from build123d import *

# Parameters (mm, degrees)
F4_T = -10
F5_R = 10


with BuildPart() as f3:
    # F0 (on Top) → F3 section 0
    with BuildSketch(Plane.XY):
        Polygon((19.5, 0), (0, 0), (-19.5, 0), (-35, -68.2623615179), (0, -68.2623615179), (35, -68.2623615179), align=None)
    # F2 (on offset) → F3 section 1
    with BuildSketch(Plane.XY.offset(-50)):
        Polygon((0, -83.2623615179), (53.7878059224, -83.2623615179), (31.4758528979, 15), (0, 15), (-31.4758528979, 15), (-53.7878059224, -83.2623615179), align=None)
    loft()

    # F4
    f4_openings = [f3.faces().sort_by_distance(p)[0] for p in [
        (0, -37.366858, 0),
        (0, -38.41676, -50),
    ]]
    offset(amount=F4_T, openings=f4_openings, kind=Kind.INTERSECTION)

    # F5
    f5_edges = [f3.edges().sort_by_distance(p)[0] for p in [
        (-25.487926, 7.5, -25),
        (-44.393903, -75.762362, -25),
        (44.393903, -75.762362, -25),
        (25.487926, 7.5, -25),
    ]]
    fillet(f5_edges, radius=F5_R)


solid = f3.part
Input: part model. Units: mm. Frame: model coordinates. A direction names the side the tool comes from. Round coordinates to 2 decimals unless told otherwise and drop trailing zeros.
1. Set-up query: faces 1 (the face through (-0.57, -67.094, -30.906)), 2 (the face through (33, -34, -50)). Return all of +Z, -Z, +X, -X, +Y, -Y with unobstructed straight access to the full face (end or side cutting, diameter ignored); none if empty.
The answers:
face 1: -Z
face 2: -Z, +X, -X, +Y, -Y
2. Pin query (flat end, axial travel): P1, Ø8, axis at x = 24.5, z = -14, coming from the +Y side; P2, Ø1, axis at y = -42, z = -23.5, coming from the -X side; P3, Ø1, axis at y = -44, z = -36, coming from the -X side. Return the tip coordinate at first contact, or that it passes through.
The answers:
P1: stops at y = 3.21
P2: stops at x = -36.46
P3: stops at x = -40.76
3. Mould query, pull axis X, two halves, no side actions, for faces 3 (the face through (0.324, -1.169, -30.906)), 4 (the face through (18, -38, 0)). Classes: released by +X, released by -X, zero draft, split by the parting line, or undercut.
The answers:
face 3: undercut
face 4: zero draft
4. Material intervals for line 1 (Y direction, x = -3.5, z = -35.5); line 2 (X direction, y = -2, z = -43); line 3 (Y direction, x = -9, z = -44), sorted ascending.
The answers:
line 1: y = -78.91 to -68.47, 0.21 to 10.65
line 2: x = -33.18 to -22.48, 22.48 to 33.18
line 3: y = -81.46 to -71.02, 2.76 to 13.2
